from build123d import *

# Parameters (mm, degrees)
SKETCH1_W           = 20
SKETCH1_H           = 40
BOSS_EXTRUDE1_DEPTH = 30


with BuildPart() as part:
    # Sketch1 → Boss-Extrude1 (new body)
    with BuildSketch(Plane(origin=(0, 0, 0), x_dir=(1, 0, 0), z_dir=(0, 1, 0))):
        Polygon((-99.811676083, 165.128212813), (-399.811676083, 165.128212813), (-399.811676083, -234.871787187), (400.188323917, -234.871787187), (400.188323917, 165.128212813), (100.188323917, 165.128212813), (50.188323917, 165.128212813), (50.188323917, 145.128212813), (50.188323917, 115.128212813), (350.188323917, 115.128212813), (350.188323917, -184.871787187), (-349.811676083, -184.871787187), (-349.811676083, 115.128212813), (-49.811676083, 115.128212813), (-49.811676083, 145.128212813), (-49.811676083, 165.128212813), align=None)
        Polygon((-99.811676083, 265.128212813), (-99.811676083, 165.128212813), (-49.811676083, 165.128212813), (-49.811676083, 185.128212813), (-49.811676083, 215.128212813), (50.188323917, 215.128212813), (50.188323917, 185.128212813), (50.188323917, 165.128212813), (100.188323917, 165.128212813), (100.188323917, 265.128212813), align=None)
        with Locations((-39.811676083, 165.128212813)):
            Rectangle(SKETCH1_W, SKETCH1_H)
        with Locations((40.188323917, 165.128212813)):
            Rectangle(SKETCH1_W, SKETCH1_H)
    extrude(amount=BOSS_EXTRUDE1_DEPTH)


solid = part.part
Source: CAD feature listing. Evaluate the final solid. Frame: model axes, mm. A direction names the side the tool comes from. Coordinates: 2 decimals unless noted, no trailing zeros. Order: outer loops, then holes, each group sorted by start corner. A loop starts at its lowest first (then second) coordinate and runs counter-clockwise, first axis right, second up. Notation, with made-up numbers: M 88.5,-15.75 L 131.5,-15.75 A34 cw 131.5,18.25 Z; hole C 13.25,71 d10. An arc over 180 degrees is marked long. Write each question's results on one line, items separated by ' | '. Start each with the question number.
Item 1: Cut plane B-B (x = -205). Return loops of the section in (y, z), and give its area (3 significant figures).
Item 2: First-contact query: pin 1 Ø1 at (x, y) = (285, 7) entering from -Z; pin 2 Ø15 at (y, z) = (16.5, -212) entering from +X; pin 3 Ø15 at (y, z) = (22, -224) entering from -X. Flat tips, straight axial feed; report the tip coordinate or a pass-through.
Item 3: Cut plane C-C (y = 16.5). Return loops of the section in (x, z), and give its area (3 significant figures).
Item 4: Set-up query: faces 1 (the face through (-202, 15, -115.128)), 2 (the face through (-5, 15, 234.872)). Return all of +Z, -Z, +X, -X, +Y, -Y with unobstructed straight access to the full face (end or side cutting, diameter ignored); none if empty.
Item 5: Draft query along X for faces 3 (the face through (100.188, 15, -214)), 4 (the face through (-31, 0, -146)), 5 (the face through (30.188, 15, -165)). Return one class per face: pulls with the +X half, pulls with the -X half, needs draft (parallel to the pull), parting line crosses it, or undercut.
Item 6: Line query: probe 1 along Z at (x, y) = (-43.5, 19); probe 2 along Z at (x, y) = (-1, 27.75); probe 3 along X at (y, z) = (16.5, -142.5). Output: solid intervals per line, ascending.
Item 7: Cut plane A-A (z = 50). Return loops of the section in (x, y), and give its area (3 significant figures).
Checked values:
1) outline: M 0,-165.13 L 30,-165.13 L 30,-115.13 L 0,-115.13 Z; M 0,184.87 L 30,184.87 L 30,234.87 L 0,234.87 Z | area: 3,000 mm2
2) pin 1: stops at z = -165.13 | pin 2: stops at x = 100.19 | pin 3: stops at x = -99.81
3) outline: M -399.81,-165.13 L -99.81,-165.13 L -99.81,-265.13 L 100.19,-265.13 L 100.19,-165.13 L 400.19,-165.13 L 400.19,234.87 L -399.81,234.87 Z; hole M -349.81,-115.13 L -49.81,-115.13 L -49.81,-145.13 L -29.81,-145.13 L -29.81,-185.13 L -49.81,-185.13 L -49.81,-215.13 L 50.19,-215.13 L 50.19,-185.13 L 30.19,-185.13 L 30.19,-145.13 L 50.19,-145.13 L 50.19,-115.13 L 350.19,-115.13 L 350.19,184.87 L -349.81,184.87 Z | area: 122,000 mm2
4) face 1: +Y, -Y | face 2: +Z, +X, -X, +Y, -Y
5) face 3: pulls with the +X half | face 4: needs draft | face 5: undercut
6) probe 1: z = -265.13 to -215.13, -185.13 to -145.13, 184.87 to 234.87 | probe 2: z = -265.13 to -215.13, 184.87 to 234.87 | probe 3: x = -399.81 to -49.81, 50.19 to 400.19
7) outline: M -399.81,0 L -349.81,0 L -349.81,30 L -399.81,30 Z; M 350.19,0 L 400.19,0 L 400.19,30 L 350.19,30 Z | area: 3,000 mm2
